from build123d import *

# Parameters (mm, degrees)
SKETCH_1_R          = 1.3
EXTRUDE_1_DEPTH     = 3
SKETCH_2_R          = 1.6
CUT_EXTRUDE_1_DEPTH = 33.790082592
CHAMFER_1_SIZE      = 0.3


with BuildPart() as part:
    # 草图1 → 凸台-拉伸1 (new body)
    with BuildSketch(Plane(origin=(0, 0, 0), x_dir=(-1, 0, 0), z_dir=(0, 0, -1))):
        with BuildLine():
            Line((8.503321513, 25.001), (-5.486589193, 25.001))
            ThreePointArc((-5.486589193, 25.001), (-14.325423958, 21.339834765), (-17.986589193, 12.501))
            Line((-17.986589193, 12.501), (-17.986589193, 12.5))
            ThreePointArc((-17.986589193, 12.5), (-14.325423958, 3.661165235), (-5.486589193, 0))
            Line((-5.486589193, 0), (8.503321493, 0))
            ThreePointArc((8.503321493, 0), (17.342156257, 3.661165235), (21.003321493, 12.5))
            ThreePointArc((21.003321493, 12.5), (17.342509831, 21.339481206), (8.503321513, 25.001))
        make_face()
        with Locations(Location((1.487905971, 21.9995, 0), (0, 0, 180))):
            Circle(SKETCH_1_R, mode=Mode.SUBTRACT)
        with Locations(Location((1.487905971, 2.9995, 0), (0, 0, 180))):
            Circle(SKETCH_1_R, mode=Mode.SUBTRACT)
        Polygon((-12.805414109, 14.989684765), (-10.744590409, 14.989684765), (-10.744590409, 18.396106406), (12.668734206, 18.396106406), (12.668734206, 5.470232129), (-10.744590409, 5.470232129), (-10.744590409, 10.001), (-12.805414109, 10.001), align=None, mode=Mode.SUBTRACT)
    extrude(amount=-EXTRUDE_1_DEPTH)

    # 草图2 → 切除-拉伸1 (cut, through all)
    with BuildSketch(Plane.XY.offset(3)):
        with Locations((-1.487905971, 21.9995)):
            Circle(SKETCH_2_R)
        with Locations((-1.487905971, 2.9995)):
            Circle(SKETCH_2_R)
    extrude(amount=-CUT_EXTRUDE_1_DEPTH, mode=Mode.SUBTRACT)

    # 倒角1
    chamfer_1_edges = [part.edges().sort_by_distance(p)[0] for p in [
        (-3.087905971, 21.9995, 0),
        (-3.087905971, 2.9995, 0),
    ]]
    chamfer(chamfer_1_edges, length=CHAMFER_1_SIZE)


solid = part.part
Verification items for the finished model (mm, model axes). A direction names the side the tool comes from. Coordinates: 2 decimals unless noted, no trailing zeros. Order: outer loops, then holes, each group sorted by start corner. A loop starts at its lowest first (then second) coordinate and runs counter-clockwise, first axis right, second up. Notation, with made-up numbers: (-38.5, 46) -> (6.5, 46) arc R29 cw to (6.5, 81) -> close; hole circle Ø11 at (15, 26.25). An arc over 180 degrees is marked (long way). Put each result on its own line as item: value. Start each with the question number.
1. Cross-section at A-A, the plane x = 4. Record the boundary of the cut face in (y, z), then the cut area to 3 significant figures.
2. Go/stop test with flat-tipped pins: pin 1 Ø1.5 at (y, z) = (7.5, 1) entering from -X; pin 2 Ø0.9 at (y, z) = (16, 2) entering from -X; pin 3 Ø1.5 at (x, z) = (-11, 1) entering from +Y. Record where each tip stops, or that it passes through.
3. Mould release check, pull along Y, two halves, no side actions. Record for faces 3 (the flat face through (-1, 0, 1)), 4 (the flat face through (-6, 21, 3)), 5 (the flat face through (-1, 18.396, 1)): released by +Y, released by -Y, zero draft, split by the parting line, or undercut.
4. Material ranges on L1, parallel to Y at x = 5.5, z = 1.15; L2, parallel to X at y = 23.25, z = 2.25; L3, parallel to X at y = 11, z = 1.1, recorded low to high. Write a range as [from, to].
5. Cross-section at B-B, the plane y = 12. Record the boundary of the cut face in (x, z), then the cut area to 3 significant figures.
6. Cross-section at C-C, the plane z = 0.9. Count the separate pieces of the cut face and the enclosed holes in it, then the cut area to 3 significant figures.
7. Access from +Z, -Z, +X, -X, +Y, -Y to the whole of each face (thin tool, end or side, straight path). Record for faces 1 (the flat face through (12, 14.99, 1)), 2 (the cylindrical face through (14.422, 3.759, 1.479)).
Computed:
1. outline: (0, 0) -> (5.47, 0) -> (5.47, 3) -> (0, 3) -> close; (18.4, 0) -> (25, 0) -> (25, 3) -> (18.4, 3) -> close
1. area: 36.2 mm2
2. pin 1: x = -20.26
2. pin 2: x = -20.63
2. pin 3: y = 24.88
3. face 3: released by -Y
3. face 4: zero draft
3. face 5: undercut
4. L1: [0, 5.47], [18.4, 25]
4. L2: [-14.88, -2.49], [-0.49, 11.87]
4. L3: [-20.91, -12.67], [12.81, 17.9]
5. outline: (-20.99, 0) -> (-12.67, 0) -> (-12.67, 3) -> (-20.99, 3) -> close; (12.81, 0) -> (17.98, 0) -> (17.98, 3) -> (12.81, 3) -> close
5. area: 40.5 mm2
6. separate pieces: 1
6. enclosed holes: 3
6. area: 512 mm2
7. face 1: +Z, -Z
7. face 2: +Z, -Z, +X, -Y
